Read the model definition and answer for the solid it produces. Units are mm, in the model's axes. A direction names the side the tool comes from. Give positions to 0.01 mm unless a question says otherwise; leave off trailing zeros. Order: outer loops, then holes, each group sorted by start corner. A loop starts at its lowest first (then second) coordinate and runs counter-clockwise, first axis right, second up. Notation, with made-up numbers: (-36, -7.75) -> (3, -7.75) arc R33 ccw to (3, 24.25) -> close; hole circle Ø2 at (26.5, 59). An arc over 180 degrees is marked (long way). Answer as CSV lines item,"result". Start each with the question number.
1) The mould has two halves that part along Z. Classify faces 1 (the face through (9.922, 6.071, -5.912)), 2 (the face through (-14, 2.5, 5)), 3 (the face through (13.343, 1.257, -6.147)), 4 (the face through (-2, 1, -1)): +Z half, -Z half, draft (parallel to the pull), parting line (faces both ways), or undercut.
2) Find section A-A (y = 8). State how many separate pieces and enclosed holes the cut face has, and give its area (3 significant figures).
3) For faces 5 (the face through (-13.343, 1.257, 6.147)), 6 (the face through (-7.5, 1, 0)), 7 (the face through (14, 2.5, -5)), determine the directions among +Z, -Z, +X, -X, +Y, -Y from which every point of the face is accessible in a straight line to the end or side of a thin tool.
4) Find section B-B (y = 4). Determine the outline of the cut face in (x, z).
5) Flat-ended cylindrical pins translate along their axes: pin 1 Ø3.5 at (x, y) = (0, 8) entering from -Z; pin 2 Ø4 at (x, y) = (10.5, 1) entering from -Z; pin 3 Ø1.3 at (x, z) = (1.33, -15.19) entering from +Y; pin 4 Ø3 at (x, z) = (4, -1.5) entering from -Y. Find the tip coordinate at first contact, or state that the pin passes through.
6) Straight lines are drawn through the part: L1, parallel to Y at x = 0, z = 11 (3 decimals); L2, parallel to X at y = 6.25, z = 0.5; L3, parallel to X at y = 8.75, z = -8.5. For each, find the intervals that lie inside material, in ascending order. Write a range as from..to.
```python
from build123d import *

# Parameters (mm, degrees)
BOSS_EXTRUDE1_DEPTH = 2
SKETCH2_R           = 13.25
BOSS_EXTRUDE2_DEPTH = 10
CUT_EXTRUDE1_DEPTH  = 8
CUT_EXTRUDE3_DEPTH  = 2
SKETCH4_R           = 1.125
CUT_EXTRUDE4_DEPTH  = 15
SKETCH5_R           = 1.125
BOSS_EXTRUDE4_DEPTH = 2.5
FILLET2_R           = 0.25
SKETCH6_W           = 1
SKETCH6_H           = 9
SKETCH6_H_2         = 14
SKETCH6_H_3         = 18
SKETCH6_H_4         = 19
SKETCH6_H_5         = 10
SKETCH6_H_6         = 6
SKETCH6_H_7         = 3
CUT_EXTRUDE5_DEPTH  = 2
FILLET3_R           = 0.25


with BuildPart() as part:
    # Sketch1 → Boss-Extrude1 (new body)
    with BuildSketch(Plane(origin=(0, 0, 0), x_dir=(1, 0, 0), z_dir=(0, 1, 0))):
        with BuildLine():
            Line((-4.094203219, 10.8), (4.094203219, 10.8))
            ThreePointArc((4.094203219, 10.8), (11.55, 0), (4.094203219, -10.8))
            Line((4.094203219, -10.8), (-4.094203219, -10.8))
            ThreePointArc((-4.094203219, -10.8), (-11.55, 0), (-4.094203219, 10.8))
        make_face()
    extrude(amount=BOSS_EXTRUDE1_DEPTH)

    # Sketch2 → Boss-Extrude2 (add)
    with BuildSketch(Plane(origin=(0, 0, 0), x_dir=(1, 0, 0), z_dir=(0, 1, 0))):
        Circle(SKETCH2_R)
        with BuildLine():
            Line((-4.094203219, -10.8), (4.094203219, -10.8))
            ThreePointArc((4.094203219, -10.8), (11.55, 0), (4.094203219, 10.8))
            Line((4.094203219, 10.8), (-4.094203219, 10.8))
            ThreePointArc((-4.094203219, 10.8), (-11.55, 0), (-4.094203219, -10.8))
        make_face(mode=Mode.SUBTRACT)
    extrude(amount=BOSS_EXTRUDE2_DEPTH)

    # Sketch3 → Cut-Extrude1 (cut)
    with BuildSketch(Plane(origin=(0, 2, 0), x_dir=(1, 0, 0), z_dir=(0, 1, 0))):
        with BuildLine():
            Line((4.094203219, -10.8), (-0.50206344, -6.943274342))
            Line((-0.50206344, -6.943274342), (7.211387877, 2.249258976))
            Line((7.211387877, 2.249258976), (11.473506452, -1.327083149))
            Line((11.473506452, -1.327083149), (12.992129547, -2.601359228))
            ThreePointArc((12.992129547, -2.601359228), (10.403847321, -8.205026564), (5.557738817, -12.02805218))
            Line((5.557738817, -12.02805218), (4.094203219, -10.8))
        make_face()
    extrude(amount=CUT_EXTRUDE1_DEPTH, mode=Mode.SUBTRACT)

    # Sketch3<3> → Cut-Extrude3 (cut)
    with BuildSketch(Plane(origin=(0, 2, 0), x_dir=(1, 0, 0), z_dir=(0, 1, 0))):
        with BuildLine():
            Line((4.094203219, -10.8), (-0.50206344, -6.943274342))
            Line((-0.50206344, -6.943274342), (7.211387877, 2.249258976))
            Line((7.211387877, 2.249258976), (11.473506452, -1.327083149))
            Line((11.473506452, -1.327083149), (12.992129547, -2.601359228))
            ThreePointArc((12.992129547, -2.601359228), (10.403847321, -8.205026564), (5.557738817, -12.02805218))
            Line((5.557738817, -12.02805218), (4.094203219, -10.8))
        make_face()
    extrude(amount=-CUT_EXTRUDE3_DEPTH, mode=Mode.SUBTRACT)

    # Sketch4 → Cut-Extrude4 (cut, symmetric)
    with BuildSketch(Plane.XY):
        with Locations((0, 8)):
            Circle(SKETCH4_R)
    extrude(amount=CUT_EXTRUDE4_DEPTH, both=True, mode=Mode.SUBTRACT)

    # Sketch5 → Boss-Extrude4 (add)
    with BuildSketch(Plane.XZ):
        with BuildLine():
            Line((3.236558978, -15.793380745), (4.260328754, -12.546397846))
            ThreePointArc((4.260328754, -12.546397846), (1.154813591, -13.19957975), (-2.016945665, -13.095588195))
            Line((-2.016945665, -13.095588195), (-0.444896589, -16.115466372))
            ThreePointArc((-0.444896589, -16.115466372), (1.503436562, -17.184358542), (3.236558978, -15.793380745))
        make_face()
        with Locations((1.329125077, -15.191969146)):
            Circle(SKETCH5_R, mode=Mode.SUBTRACT)
        with BuildLine():
            Line((15.947891709, -2.360283757), (13.246875724, -0.287721297))
            ThreePointArc((13.246875724, -0.287721297), (12.798517198, -3.429352348), (11.615991547, -6.37426391))
            Line((11.615991547, -6.37426391), (14.991421235, -5.929880161))
            ThreePointArc((14.991421235, -5.929880161), (16.662220503, -4.464628528), (15.947891709, -2.360283757))
        make_face()
        with Locations((14.730368851, -3.946990438)):
            Circle(SKETCH5_R, mode=Mode.SUBTRACT)
        with BuildLine():
            Line((-3.236558978, 15.793380745), (-4.260328754, 12.546397846))
            ThreePointArc((-4.260328754, 12.546397846), (-1.154813591, 13.19957975), (2.016945665, 13.095588195))
            Line((2.016945665, 13.095588195), (0.444896589, 16.115466372))
            ThreePointArc((0.444896589, 16.115466372), (-1.503436562, 17.184358542), (-3.236558978, 15.793380745))
        make_face()
        with Locations((-1.329125077, 15.191969146)):
            Circle(SKETCH5_R, mode=Mode.SUBTRACT)
        with BuildLine():
            Line((-15.947891709, 2.360283757), (-13.246875724, 0.287721297))
            ThreePointArc((-13.246875724, 0.287721297), (-12.798517198, 3.429352348), (-11.615991547, 6.37426391))
            Line((-11.615991547, 6.37426391), (-14.991421235, 5.929880161))
            ThreePointArc((-14.991421235, 5.929880161), (-16.662220503, 4.464628528), (-15.947891709, 2.360283757))
        make_face()
        with Locations((-14.730368851, 3.946990438)):
            Circle(SKETCH5_R, mode=Mode.SUBTRACT)
    extrude(amount=-BOSS_EXTRUDE4_DEPTH)

    # Fillet2
    fillet2_edges = [part.edges().sort_by_distance(p)[0] for p in [
        (-1.154813591, 2.5, 13.19957975),
        (2.016945665, 1.25, 13.095588195),
        (-4.260328754, 1.25, 12.546397846),
        (-12.798517198, 2.5, 3.429352348),
        (-11.615991547, 1.25, 6.37426391),
        (-13.246875724, 1.25, 0.287721297),
        (0, 2, -10.8),
        (9.866860318, 2, -6.003962647),
        (-11.55, 2, 0),
        (-0.50206344, 1, 6.943274342),
        (7.211387877, 1, -2.249258976),
        (1.154813591, 2.5, -13.19957975),
        (-2.016945665, 1.25, -13.095588195),
        (4.260328754, 1.25, -12.546397846),
        (0, 2, 10.8),
        (12.798517198, 2.5, -3.429352348),
        (11.615991547, 1.25, -6.37426391),
        (13.246875724, 1.25, -0.287721297),
    ]]
    fillet(fillet2_edges, radius=FILLET2_R)

    # Sketch6 → Cut-Extrude5 (cut)
    with BuildSketch(Plane.XZ):
        with Locations((-9.25, -0.40318756)):
            Rectangle(SKETCH6_W, SKETCH6_H)
        with Locations((-7, -0.119489057)):
            Rectangle(SKETCH6_W, SKETCH6_H_2)
        with Locations((-4.75, -0.183989082)):
            Rectangle(SKETCH6_W, SKETCH6_H_3)
        with Locations((-2.5, -0.407091801)):
            Rectangle(SKETCH6_W, SKETCH6_H_4)
        with Locations((-0.25, -2.730474383)):
            Rectangle(SKETCH6_W, SKETCH6_H_2)
        with Locations((2, -3.212459658)):
            Rectangle(SKETCH6_W, SKETCH6_H_5)
        with Locations((4.25, -3.573003756)):
            Rectangle(SKETCH6_W, SKETCH6_H_6)
        with Locations((6.5, -4.222915511)):
            Rectangle(SKETCH6_W, SKETCH6_H_7)
    extrude(amount=-CUT_EXTRUDE5_DEPTH, mode=Mode.SUBTRACT)

    # Fillet3
    fillet3_edges = [part.edges().sort_by_distance(p)[0] for p in [
        (-8.75, 1, -4.90318756),
        (-8.75, 1, 4.09681244),
        (-9.75, 1, 4.09681244),
        (-9.75, 1, -4.90318756),
        (-6.5, 1, -7.119489057),
        (-6.5, 1, 6.880510943),
        (-7.5, 1, 6.880510943),
        (-7.5, 1, -7.119489057),
        (-4.25, 1, -9.183989082),
        (-4.25, 1, 8.816010918),
        (-5.25, 1, 8.816010918),
        (-5.25, 1, -9.183989082),
        (-2, 1, -9.907091801),
        (-2, 1, 9.092908199),
        (-3, 1, 9.092908199),
        (-3, 1, -9.907091801),
        (0.25, 1, -9.730474383),
        (0.25, 1, 4.269525617),
        (-0.75, 1, 4.269525617),
        (-0.75, 1, -9.730474383),
        (2.5, 1, -8.212459658),
        (2.5, 1, 1.787540342),
        (1.5, 1, 1.787540342),
        (1.5, 1, -8.212459658),
        (4.75, 1, -6.573003756),
        (4.75, 1, -0.573003756),
        (3.75, 1, -0.573003756),
        (3.75, 1, -6.573003756),
        (7, 1, -5.722915511),
        (7, 1, -2.722915511),
        (6, 1, -2.722915511),
        (6, 1, -5.722915511),
    ]]
    fillet(fillet3_edges, radius=FILLET3_R)


solid = part.part
```
Findings below:
1,face 1,"undercut"
1,face 2,"draft"
1,face 3,"-Z half"
1,face 4,"undercut"
2,separate pieces,"3"
2,enclosed holes,"0"
2,area,"108 mm²"
3,face 5,"+Z, -X, +Y, -Y"
3,face 6,"+Y, -Y"
3,face 7,"-Z, +X, +Y"
4,outline,"(-4.09, -10.8) arc R11.55 cw to (-4.09, 10.8) -> (4.09, 10.8) -> (5.56, 12.03) arc R13.25 ccw (long way) to (12.99, 2.6) -> (11.47, 1.33) arc R11.55 cw to (4.09, -10.8) -> close"
5,pin 1,"z = -13.25"
5,pin 2,"z = -10.16"
5,pin 3,"through"
5,pin 4,"y = 0"
6,L1,"0..6.875, 9.125..10"
6,L2,"-13.24..-11.54, 11.54..13.24"
6,L3,"-10.16..-7.82, 7.82..10.16"
